Work out the finished part from the listing and answer in its coordinate system (mm). Face numbers are marked on the shaded views. A direction names the side the tool comes from. Round coordinates to 2 decimals unless told otherwise and drop trailing zeros. Order: outer loops, then holes, each group sorted by start corner. A loop starts at its lowest first (then second) coordinate and runs counter-clockwise, first axis right, second up. Notation, with made-up numbers: (8, 44) - (38, 44) arc R12 cw to (38, 62) - close; hole circle Ø4 at (47.25, 27.5). An arc over 180 degrees is marked (long way). Use one line per item in the form item = value. Start each with the question number.
Q1. Find the intervals of material crossed by line 1 (X direction, y = 1.5, z = -0.1); line 2 (Z direction, x = 4.95, y = 18); line 3 (X direction, y = 18.5, z = 2.75), in increasing order. Write a range as [from, to].
Q2. The part is cut by section B-B on x = -7.5. Determine the outline of the cut face in (y, z).
Q3. For a pull along X with two mould halves and no side action, classify the marked faces 1, 2, 3 and 4 as +X half, -X half, draft (parallel to the pull), parting line (faces both ways), or undercut.
Q4. Which of the six approach directions +Z, -Z, +X, -X, +Y, -Y give full straight-line access (tool end or side, diameter ignored) to the marked faces 5, 6 and 7?
Q5. The part is cut by section A-A on z = 1.1. Determine the outline of the cut face in (x, y), plus the area to 3 significant figures.
Q6. Given P1, Ø3, axis at y = 10, z = 0, coming from the +X side; P2, Ø1.5, axis at x = -1, z = -2, coming from the +Y side; P3, Ø2, axis at x = -7, z = -0.5, coming from the +Y side; P4, Ø1.5, axis at x = 3.5, z = -1, coming from the +Y side, each flat-ended and moving along its own axis, determine where each tip first touches the part or whether it passes through.
Q7. The part is cut by section C-C on y = 11.5. Determine the outline of the cut face in (x, z).
Q8. The part is cut by section D-D on z = 0. Determine the outline of the cut face in (x, y), plus the area to 3 significant figures.
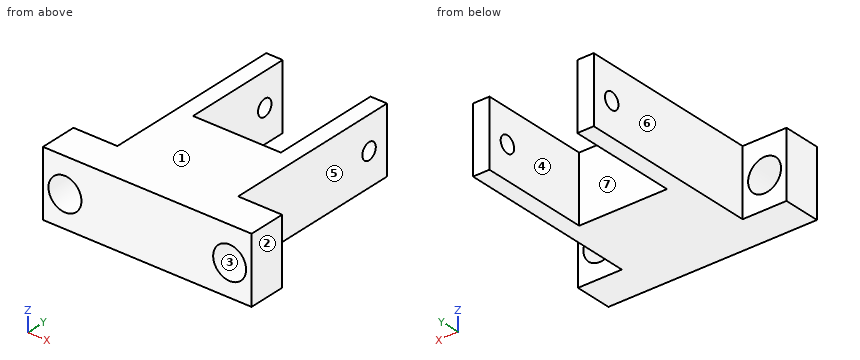
from build123d import *

# Parameters (mm, degrees)
SKETCH1_R               = 1.5
BOSS_EXTRUDE1_DEPTH     = 3.4
SKETCH1_4_W             = 1.5
SKETCH1_4_H             = 6
BOSS_EXTRUDE2_DEPTH     = 20
CUT_EXTRUDE1_DEPTH      = 26.179356624
CUT_EXTRUDE1_DEPTH_BACK = 26.179356624
SKETCH2_R               = 0.75
SKETCH1_5_W             = 8
SKETCH1_5_H             = 6
BOSS_EXTRUDE3_DEPTH     = 10


with BuildPart() as part:
    # Sketch1 → Boss-Extrude1 (new body)
    with BuildSketch(Plane(origin=(0, 0, 0), x_dir=(1, 0, 0), z_dir=(0, 1, 0))):
        Polygon((-9.5, 3), (-9.5, -3), (9.5, -3), (9.5, 3), (0, 3), align=None)
        with Locations(Location((-7.5, 0.128979829, 0), (0, 0, 270))):
            Circle(SKETCH1_R, mode=Mode.SUBTRACT)
        with Locations(Location((7.5, 0.128979829, 0), (0, 0, 270))):
            Circle(SKETCH1_R, mode=Mode.SUBTRACT)
    extrude(amount=BOSS_EXTRUDE1_DEPTH)

    # Sketch1_4 → Boss-Extrude2 (add)
    with BuildSketch(Plane(origin=(0, 0, 0), x_dir=(1, 0, 0), z_dir=(0, 1, 0))):
        with Locations((-4.75, 0)):
            Rectangle(SKETCH1_4_W, SKETCH1_4_H)
        with Locations((4.75, 0)):
            Rectangle(SKETCH1_4_W, SKETCH1_4_H)
    extrude(amount=BOSS_EXTRUDE2_DEPTH)

    # Sketch2 → Cut-Extrude1 (cut, two sides: drawn at the far end of the back side and taken through both)
    with BuildSketch(Plane(origin=(5.5, 0, 0), x_dir=(0, 0, -1), z_dir=(1, 0, 0)).offset(-CUT_EXTRUDE1_DEPTH_BACK)):
        with Locations((0, 18)):
            Circle(SKETCH2_R)
    extrude(amount=CUT_EXTRUDE1_DEPTH + CUT_EXTRUDE1_DEPTH_BACK, mode=Mode.SUBTRACT)

    # Sketch1_5 → Boss-Extrude3 (add)
    with BuildSketch(Plane(origin=(0, 0, 0), x_dir=(1, 0, 0), z_dir=(0, 1, 0))):
        Rectangle(SKETCH1_5_W, SKETCH1_5_H)
    extrude(amount=BOSS_EXTRUDE3_DEPTH)


solid = part.part
Found:
q1.line_1 = [-9.5, -9], [-6, 6], [9, 9.5]
q1.line_2 = [-3, -0.75], [0.75, 3]
q1.line_3 = [-5.5, -4], [4, 5.5]
q2.outline = (0, -3) - (3.4, -3) - (3.4, -1.63) - (0, -1.63) - close; (0, 1.37) - (3.4, 1.37) - (3.4, 3) - (0, 3) - close
q3.face_1 = draft
q3.face_2 = +X half
q3.face_3 = undercut
q3.face_4 = undercut
q4.face_5 = +Z, -Z, +X, +Y
q4.face_6 = +Z, -Z, -X, +Y
q4.face_7 = +Z, -Z, +Y
q5.outline = (-9.5, 0) - (-8.36, 0) - (-8.36, 3.4) - (-9.5, 3.4) - close; (-6.64, 0) - (6.64, 0) - (6.64, 3.4) - (5.5, 3.4) - (5.5, 20) - (4, 20) - (4, 10) - (-4, 10) - (-4, 20) - (-5.5, 20) - (-5.5, 3.4) - (-6.64, 3.4) - close; (8.36, 0) - (9.5, 0) - (9.5, 3.4) - (8.36, 3.4) - close
q5.area = 156 mm²
q6.P1 = 5.5
q6.P2 = 10
q6.P3 = 3.4
q6.P4 = 20
q7.outline = (-5.5, -3) - (-4, -3) - (-4, 3) - (-5.5, 3) - close; (4, -3) - (5.5, -3) - (5.5, 3) - (4, 3) - close
q8.outline = (-9.5, 0) - (-8.99, 0) - (-8.99, 3.4) - (-9.5, 3.4) - close; (-6.01, 0) - (6.01, 0) - (6.01, 3.4) - (5.5, 3.4) - (5.5, 17.25) - (4, 17.25) - (4, 10) - (-4, 10) - (-4, 17.25) - (-5.5, 17.25) - (-5.5, 3.4) - (-6.01, 3.4) - close; (-5.5, 18.75) - (-4, 18.75) - (-4, 20) - (-5.5, 20) - close; (4, 18.75) - (5.5, 18.75) - (5.5, 20) - (4, 20) - close; (8.99, 0) - (9.5, 0) - (9.5, 3.4) - (8.99, 3.4) - close
q8.area = 142 mm²
